Design review of the part built by this model. Coordinates are the model's own, in mm. A direction names the side the tool comes from. Coordinates: 2 decimals unless noted, no trailing zeros. Write each loop counter-clockwise with the first axis right and the second up, starting at its lowest first coordinate (ties: lowest second). Pieces come first, ordered by that corner, then holes.
Q1. For probe 1 along Y at (x, z) = (25, 6); probe 2 along X at (y, z) = (22, 5.75) (3 decimals); probe 3 along X at (y, z) = (12, 0) (3 decimals), list the stretches that pass through material, from the lowest coordinate up.
Q2. Take a section at D-D (x = -55). Give the boundary of the cut face in (y, z).
Q3. Take a section at C-C (z = -4.75). Give the boundary of the cut face in (x, y) (3 decimals), and give its area (3 significant figures).
Q4. Take a section at B-B (y = 1). Give the boundary of the cut face in (x, z) (1 decimal), and give its area (3 significant figures).
Q5. Mouldability with a two-part tool opening along X and no side actions: class faces 4 (the flat face through (40.05, -1.61, 0.11)), 5 (the flat face through (16, 19.05, 0)), 6 (the flat face through (19, 0, 0)) as pulls with the +X half, pulls with the -X half, needs draft (parallel to the pull), parting line crosses it, or undercut.
Q6. Machinability: for faces 1 (the flat face through (28, -6.35, 0)), 2 (the flat face through (0, 9, 0)), 3 (the flat face through (38.03, 15.83, 0.11)), which of the approach directions +Z, -Z, +X, -X, +Y, -Y give a long, thin tool a straight path to every point of the face, cutting with its end or side? Answer none if there is none.
Q7. Take a section at A-A (x = 9). Give the boundary of the cut face in (y, z), and give its area (3 significant figures).
Q8. Insertion check: pin 1 (3 mm diameter, centred on x = -26, z = 1.5, fed in from -Y); pin 2 (8 mm diameter, centred on x = 23, z = -1.5, fed in from -Y); pin 3 (8 mm diameter, centred on y = 13, z = -3.5, fed in from +X); pin 4 (2 mm diameter, centred on x = -12, y = 9.5, fed in from +Z). Each pin has a flat end and moves straight along its axis. Give the tip position at first contact, or say it passes through.
```python
from build123d import *

# Parameters (mm, degrees)
F0_DEPTH = 7.9375
F1_R     = 19.05


with BuildPart() as f0:
    # F2 (on Top) → F0 (new body, symmetric)
    with BuildSketch(Plane.XY):
        with BuildLine():
            Line((36.83, 0), (0, 0))
            Line((0, 0), (0, 19.05))
            Line((0, 19.05), (33.02, 19.05))
            Line((33.02, 19.05), (33.02, 12.7))
            Line((33.02, 12.7), (43.18, 19.05))
            Line((43.18, 19.05), (43.18, 25.4))
            Line((43.18, 25.4), (-9.525, 25.4))
            Line((-9.525, 25.4), (-9.525, -6.35))
            ThreePointArc((-9.525, -6.35), (-30.491958, -22.48979), (-52.311708, -7.523005))
            ThreePointArc((-52.311708, -7.523005), (-53.687003, 3.104461), (-62.729088, -2.646641))
            ThreePointArc((-62.729088, -2.646641), (-62.723566, -2.872597), (-62.707014, -3.098013))
            ThreePointArc((-62.707014, -3.098013), (-32.752866, -31.707391), (0, -6.35))
            Line((0, -6.35), (43.18, -6.35))
            Line((43.18, -6.35), (43.18, -3.175))
            Line((43.18, -3.175), (36.83, 0))
        make_face()
    extrude(amount=F0_DEPTH, both=True)

    # F1
    f1_edges = [f0.edges().sort_by_distance(p)[0] for p in [
        (0, -6.35, 0),
    ]]
    fillet(f1_edges, radius=F1_R)


solid = f0.part
```
Response:
1. probe 1: y = -6.35 to 0, 19.05 to 25.4
1. probe 2: x = -9.525 to 43.18
1. probe 3: x = -9.525 to 0
2. outline: (-20.91, -7.94) - (3.55, -7.94) - (3.55, 7.94) - (-20.91, 7.94) - close
3. outline: (-62.729, -2.647) arc R4.626 ccw to (-62.707, -3.098) arc R31.75 ccw to (-3.612, -15.875) arc R19.05 cw to (12.886, -6.35) - (43.18, -6.35) - (43.18, -3.175) - (36.83, 0) - (0, 0) - (0, 19.05) - (33.02, 19.05) - (33.02, 12.7) - (43.18, 19.05) - (43.18, 25.4) - (-9.525, 25.4) - (-9.525, -6.35) arc R22.498 cw to (-52.312, -7.523) arc R6.35 ccw (long way) to start
3. area: 1,680 mm2
4. outline: (-61.6, -7.9) - (-51.2, -7.9) - (-51.2, 7.9) - (-61.6, 7.9) - close; (-9.5, -7.9) - (0, -7.9) - (0, 7.9) - (-9.5, 7.9) - close
4. area: 316 mm2
5. face 4: pulls with the +X half
5. face 5: undercut
5. face 6: needs draft
6. face 1: +Z, -Z, +X, -Y
6. face 2: +Z, -Z
6. face 3: +Z, -Z, +X
7. outline: (-6.75, -7.94) - (0, -7.94) - (0, 7.94) - (-6.75, 7.94) - close; (19.05, -7.94) - (25.4, -7.94) - (25.4, 7.94) - (19.05, 7.94) - close
7. area: 208 mm2
8. pin 1: stops at y = -31.54
8. pin 2: stops at y = -6.35
8. pin 3: stops at x = 39.9
8. pin 4: passes through
